Here's the drawing with two shaded views (mm, measured from the low corner). I have some questions. A direction names the side the tool comes from. Give positions to 0.01 mm unless a question says otherwise; leave off trailing zeros. Write each loop counter-clockwise with the first axis right and the second up, starting at its lowest first coordinate (ties: lowest second). Pieces come first, ordered by that corner, then holes. Notation, with made-up numbers: M 23.25,-31.75 L 44.25,-31.75 A17 cw 44.25,-25.75 Z; hole C -19,61.5 d7. An arc over 180 degrees is marked long. Answer as CSV lines item,"result". Start each with the question number.
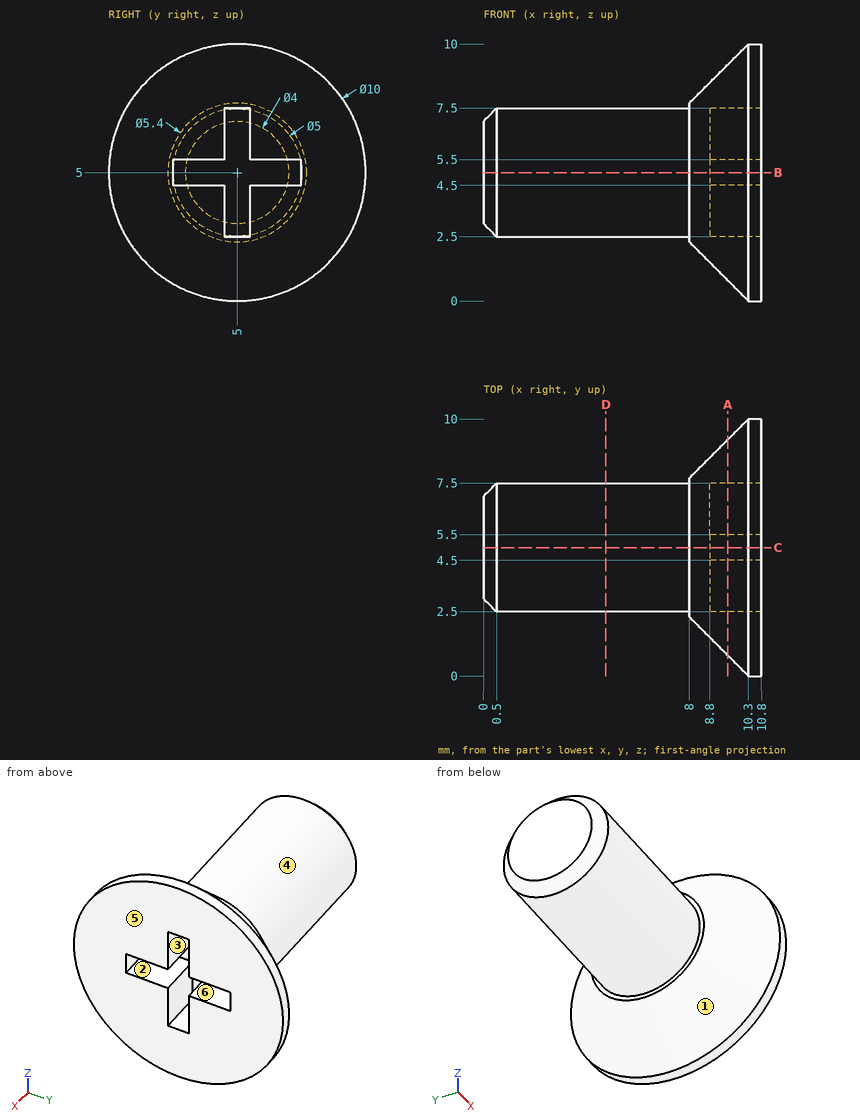
1. Imagine slicing it at A-A, the plane x = 9.5. Please give me the cut outline in (y, z), plus the area to 3 significant figures.
2. Thinking about a two-plate mould opening in Y: for the marked faces 3, 4, 5 and 6, which applies, pulls with the +Y half, pulls with the -Y half, needs draft (parallel to the pull), parting line crosses it, or undercut?
3. Please list where these lines run through material, in increasing order: line 1 (Z direction, x = 10.25, y = 4); line 2 (X direction, y = 5.25, z = 5); line 3 (X direction, y = 3, z = 8.25).
4. On a 3-axis mill with a long thin cutter (end or side, diameter ignored), from which of +Z, -Z, +X, -X, +Y, -Y can I reach the whole of each face in a straight line? I mean the marked faces 1 and 2. Say none if no direction works.
5. Imagine slicing it at D-D, the plane x = 4.75. Please give me the cut outline in (y, z).
6. Imagine slicing it at B-B, the plane z = 5. Please give me the cut outline in (x, y), plus the area to 3 significant figures.
7. Will these pins go through, and if not, where does the flat tip stop? P1, Ø0.6, axis at x = 9.5, y = 3.5, coming from the -Z side; P2, Ø0.5, axis at x = 9.5, y = 5, coming from the +Z side; P3, Ø2, axis at x = 10, y = 3, coming from the +Z side.
Solutions:
1,outline,"C 5,5 d8.4; hole M 2.5,4.5 L 4.5,4.5 L 4.5,2.5 L 5.5,2.5 L 5.5,4.5 L 7.5,4.5 L 7.5,5.5 L 5.5,5.5 L 5.5,7.5 L 4.5,7.5 L 4.5,5.5 L 2.5,5.5 Z"
1,area,"46.4 mm²"
2,face 3,"undercut"
2,face 4,"parting line crosses it"
2,face 5,"needs draft"
2,face 6,"undercut"
3,line 1,"0.15 to 4.5, 5.5 to 9.85"
3,line 2,"0 to 8.8"
3,line 3,"9.12 to 10.8"
4,face 1,"-X"
4,face 2,"+X"
5,outline,"C 5,5 d5"
6,outline,"M 0,3 L 0.5,2.5 L 8,2.5 L 8,2.3 L 10.3,0 L 10.8,0 L 10.8,2.5 L 8.8,2.5 L 8.8,7.5 L 10.8,7.5 L 10.8,10 L 10.3,10 L 8,7.7 L 8,7.5 L 0.5,7.5 L 0,7 Z"
6,area,"52.5 mm²"
7,P1,"z = 0.74"
7,P2,"z = 9.45"
7,P3,"z = 9.89"
